Input: part model. Units: mm. Frame: model coordinates. A direction names the side the tool comes from. Round coordinates to 2 decimals unless told otherwise and drop trailing zeros. Loops run counter-clockwise (first coordinate to the right, second up) from the corner with the lowest first, then second, coordinate; pieces in that order, holes last. Notation, with made-up numbers: (38, 20.25) -> (83, 20.25) arc R22 ccw to (83, 50.25) -> close; hole circle Ø11 at (68, 85). An arc over 180 degrees is marked (long way). Answer as a JSON object with one key per item and string values.
```python
from build123d import *

# Parameters (mm, degrees)
F0_W     = 9
F0_H     = 9
F0_R     = 3
F0_R_2   = 18
F0_R_3   = 9
F0_R_4   = 4.5
F1_DEPTH = 10


with BuildPart() as f1:
    # F0 (on Top) → F1 (new body)
    with BuildSketch(Plane.XY):
        Polygon((49.276882, 69.50716), (-69.223118, 69.50716), (-69.223118, -78.99284), (-19.723118, -78.99284), (-19.723118, -53.49284), (49.276882, -53.49284), align=None)
        with Locations((-60.223118, -67.803344)):
            Rectangle(F0_W, F0_H, mode=Mode.SUBTRACT)
        with Locations((-43.723118, -67.803344)):
            Rectangle(F0_W, F0_H, mode=Mode.SUBTRACT)
        with Locations((-60.223118, -45.303344)):
            Circle(F0_R, mode=Mode.SUBTRACT)
        with Locations((-28.723118, -67.803344)):
            Rectangle(F0_W, F0_H, mode=Mode.SUBTRACT)
        with Locations((-36.221969, -16.99284)):
            Circle(F0_R_2, mode=Mode.SUBTRACT)
        with Locations((40.278031, -42.957689)):
            Circle(F0_R, mode=Mode.SUBTRACT)
        with Locations((2.778031, -16.99284)):
            Circle(F0_R_3, mode=Mode.SUBTRACT)
        with Locations((28.278031, -16.99284)):
            Circle(F0_R_3, mode=Mode.SUBTRACT)
        with Locations((-31.781744, 17.50716)):
            Circle(F0_R, mode=Mode.SUBTRACT)
        with BuildLine():
            Line((-54.223118, 27.50716), (-54.223118, 51.50716))
            Line((-54.223118, 51.50716), (-30.223118, 51.50716))
            ThreePointArc((-30.223118, 51.50716), (-26.473118, 47.75716), (-30.223118, 44.00716))
            Line((-30.223118, 44.00716), (-46.723118, 44.00716))
            Line((-46.723118, 44.00716), (-46.723118, 27.50716))
            Line((-46.723118, 27.50716), (-54.223118, 27.50716))
        make_face(mode=Mode.SUBTRACT)
        with Locations((-60.223118, 60.50716)):
            Circle(F0_R, mode=Mode.SUBTRACT)
        with BuildLine():
            Line((-9.223118, 14.00716), (-9.223118, 32.00716))
            ThreePointArc((-9.223118, 32.00716), (-3.223118, 38.00716), (2.776882, 32.00716))
            Line((2.776882, 32.00716), (2.776882, 14.00716))
            ThreePointArc((2.776882, 14.00716), (-3.223118, 8.00716), (-9.223118, 14.00716))
        make_face(mode=Mode.SUBTRACT)
        with Locations((20.23034, 17.50716)):
            Circle(F0_R, mode=Mode.SUBTRACT)
        with Locations((31.014569, 17.50716)):
            Circle(F0_R_4, mode=Mode.SUBTRACT)
        with Locations((39.73034, 60.50716)):
            Circle(F0_R, mode=Mode.SUBTRACT)
    extrude(amount=F1_DEPTH)


solid = f1.part
```
1) Section A-A, the plane y = 29.5. Output: boundary loops of the cut face in (x, z).
Output:
{"outline": "(-69.22, 0) -> (-54.22, 0) -> (-54.22, 10) -> (-69.22, 10) -> close; (-46.72, 0) -> (-9.22, 0) -> (-9.22, 10) -> (-46.72, 10) -> close; (2.78, 0) -> (49.28, 0) -> (49.28, 10) -> (2.78, 10) -> close"}
2) Ray query, probe 1 along X at (y, z) = (-69, 4.75); probe 2 along X at (y, z) = (37, 7.5); probe 3 along X at (y, z) = (-22.5, 2). Return the intervals inside material, ascending.
Output:
{"probe 1": "x = -69.22 to -64.72, -55.72 to -48.22, -39.22 to -33.22, -24.22 to -19.72", "probe 2": "x = -69.22 to -54.22, -46.72 to -6.55, 0.1 to 49.28", "probe 3": "x = -69.22 to -53.36, -19.09 to -4.34, 9.9 to 21.16, 35.4 to 49.28"}
3) Reachability of faces 3 (the face through (-9, 69.507, 5)), 4 (the face through (-24.223, -68, 5)) from +Z, -Z, +X, -X, +Y, -Y: full face, straight path, thin tool, end or side. Return the list, or none.
Output:
{"face 3": "+Z, -Z, +X, -X, +Y", "face 4": "+Z, -Z"}
4) Draft query along X for faces 1 (the face through (27.444, 14.769, 4.93)), 2 (the face through (-11, -4, 0)). Return one class per face: +X half, -X half, draft (parallel to the pull), parting line (faces both ways), or undercut.
Output:
{"face 1": "undercut", "face 2": "draft"}
5) Contact query for flat-ended pins moving along their axis: P1, Ø16, axis at x = 28.28, y = -16.99, coming from the +Z side; P2, Ø3, axis at x = 21.5, z = 5, coming from the -Y side. Output: stop coordinate, or through.
Output:
{"P1": "passes through", "P2": "stops at y = -53.49"}
6) Section D-D, the plane y = -61. Output: boundary loops of the cut face in (x, z).
Output:
{"outline": "(-69.22, 0) -> (-19.72, 0) -> (-19.72, 10) -> (-69.22, 10) -> close"}
7) Section C-C, the plane x = -41. Output: boundary loops of the cut face in (y, z).
Output:
{"outline": "(-78.99, 0) -> (-72.3, 0) -> (-72.3, 10) -> (-78.99, 10) -> close; (-63.3, 0) -> (-34.35, 0) -> (-34.35, 10) -> (-63.3, 10) -> close; (0.36, 0) -> (44.01, 0) -> (44.01, 10) -> (0.36, 10) -> close; (51.51, 0) -> (69.51, 0) -> (69.51, 10) -> (51.51, 10) -> close"}
8) Section B-B, the plane x = 10. Output: boundary loops of the cut face in (y, z).
Output:
{"outline": "(-53.49, 0) -> (-22.36, 0) -> (-22.36, 10) -> (-53.49, 10) -> close; (-11.62, 0) -> (69.51, 0) -> (69.51, 10) -> (-11.62, 10) -> close"}
